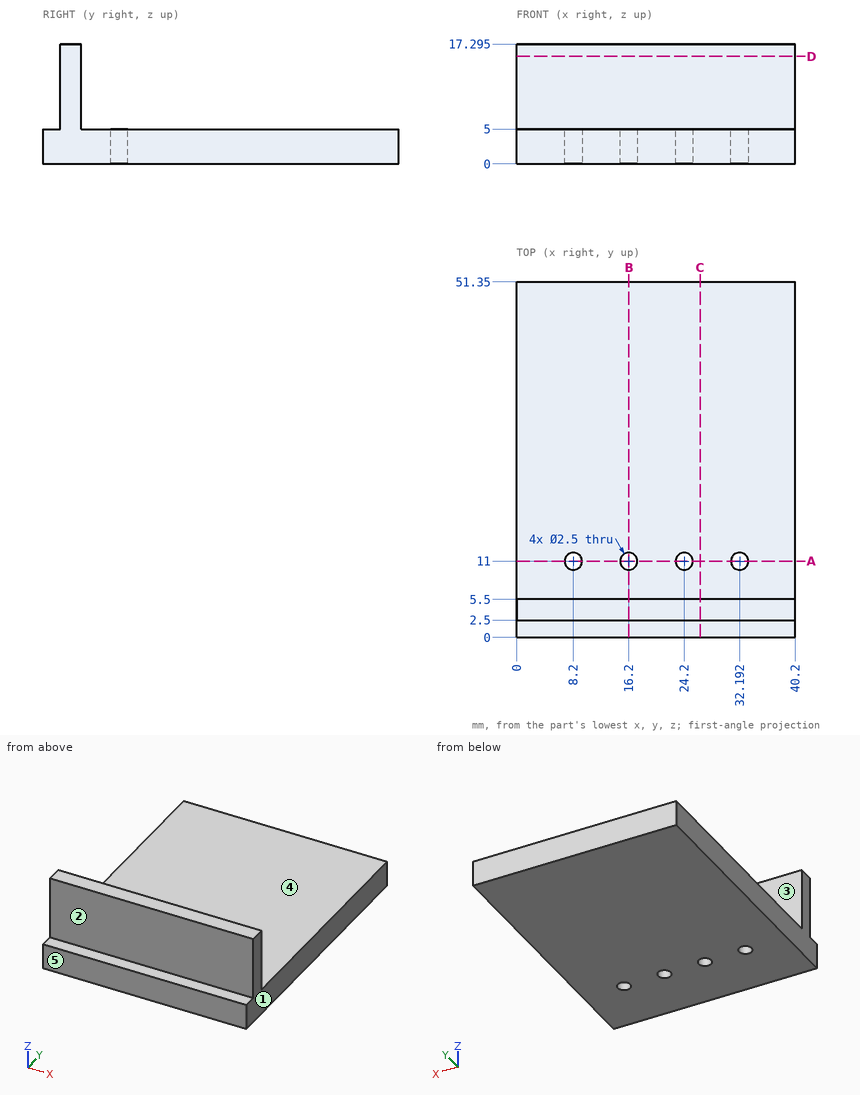
Here's the drawing with two shaded views (mm, measured from the low corner). I have some questions. A direction names the side the tool comes from. Give positions to 0.01 mm unless a question says otherwise; leave off trailing zeros. Loops run counter-clockwise (first coordinate to the right, second up) from the corner with the lowest first, then second, coordinate; pieces in that order, holes last. Notation, with made-up numbers: M 9,65 L 37,65 A23 ccw 37,99 Z; hole C 14,54 d10. An arc over 180 degrees is marked long. One line per item, written item: value.
(1) I need wall thicknesses on line 1 (Y direction, x = 24.2, z = 1.1); line 2 (Y direction, x = 23, z = 12.5); line 3 (Z direction, x = 3, y = 35.5). Which ranges of each line are inside material? Lowest first, please.
Returned:
line 1: 0 to 9.75, 12.25 to 51.35
line 2: 2.5 to 5.5
line 3: 0 to 5
(2) Suppose I cut it at D-D on z = 15.5. List the corners of the cut face in (x, y) for me.
Returned:
outline: M 0,2.5 L 40.2,2.5 L 40.2,5.5 L 0,5.5 Z
(3) Will these pins go through, and if not, where does the flat tip stop? pin 1 (2 mm diameter, centred on x = 24.2, y = 11, fed in from -Z); pin 2 (1.5 mm diameter, centred on y = 6, z = 11.5, fed in from +X); pin 3 (1.5 mm diameter, centred on x = 30, y = 9.5, fed in from +Z); pin 4 (6 mm diameter, centred on x = 19, z = 12.5, fed in from -Y).
Returned:
pin 1: through
pin 2: x = 40.2
pin 3: z = 5
pin 4: y = 2.5
(4) We'd pull the mould along Y, two halves only. Please class the marked faces 1, 2 and 3: released by +Y, released by -Y, zero draft, split by the parting line, or undercut.
Returned:
face 1: zero draft
face 2: released by -Y
face 3: released by +Y
(5) Suppose I cut it at C-C on x = 26.5. List the corners of the cut face in (y, z) for me (3 decimals).
Returned:
outline: M 0,0 L 51.35,0 L 51.35,5 L 5.5,5 L 5.5,17.295 L 2.5,17.295 L 2.5,5 L 0,5 Z
(6) Which directions (+Z, -Z, +X, -X, +Y, -Y) give clear straight access to the entire face, cutting with the end or side of a thin tool? Please do the marked faces 4 and 5.
Returned:
face 4: +Z, +X, -X, +Y
face 5: +Z, -Z, +X, -X, -Y
(7) Suppose I cut it at A-A on y = 11. List the corners of the cut face in (x, z) for me.
Returned:
outline: M 0,0 L 6.95,0 L 6.95,5 L 0,5 Z; M 9.45,0 L 14.95,0 L 14.95,5 L 9.45,5 Z; M 17.45,0 L 22.95,0 L 22.95,5 L 17.45,5 Z; M 25.45,0 L 30.94,0 L 30.94,5 L 25.45,5 Z; M 33.44,0 L 40.2,0 L 40.2,5 L 33.44,5 Z
(8) Suppose I cut it at B-B on x = 16.2. List the corners of the cut face in (y, z) for me (3 decimals), plus the area to 3 significant figures.
Returned:
outline: M 0,0 L 9.75,0 L 9.75,5 L 5.5,5 L 5.5,17.295 L 2.5,17.295 L 2.5,5 L 0,5 Z; M 12.25,0 L 51.35,0 L 51.35,5 L 12.25,5 Z
area: 281 mm^2
